```python
from build123d import *

# Parameters (mm, degrees)
SKETCH1_W           = 390
SKETCH1_H           = 88
BOSS_EXTRUDE1_DEPTH = 60
SKETCH2_R           = 13.520117845
BOSS_EXTRUDE2_DEPTH = 10
LPATTERN1_COUNT     = 6
LPATTERN1_PITCH     = 60


with BuildPart() as part:
    # Sketch1 → Boss-Extrude1 (new body)
    with BuildSketch(Plane.XY):
        with Locations((2.535, 19.375)):
            Rectangle(SKETCH1_W, SKETCH1_H)
    extrude(amount=BOSS_EXTRUDE1_DEPTH)

    # Sketch2 → Boss-Extrude2 (add)
    with BuildSketch(Plane.XY.offset(60)):
        with Locations((-142.569495457, 17.704999413)):
            Circle(SKETCH2_R)
    boss_extrude2 = extrude(amount=BOSS_EXTRUDE2_DEPTH)

    # LPattern1: Boss-Extrude2 ×6
    with Locations(*[(i * LPATTERN1_PITCH, 0, 0) for i in range(1, LPATTERN1_COUNT)]):
        add(boss_extrude2)


solid = part.part
```
For this review, take the finished solid that the model builds, in its own axes (mm). A direction names the side the tool comes from. Round coordinates to 2 decimals unless told otherwise and drop trailing zeros. Write each loop counter-clockwise with the first axis right and the second up, starting at its lowest first coordinate (ties: lowest second). Pieces come first, ordered by that corner, then holes. Notation, with made-up numbers: (56, 48.5) - (68, 48.5) arc R21 ccw to (68, 83.5) - close; hole circle Ø4 at (56.25, 60.25). An arc over 180 degrees is marked (long way). Answer as a JSON object with one key per item and string values.
1. We need section D-D on y = 23.5. Give the boundary of the cut face in (x, z) (3 decimals), then the cut area to 3 significant figures.
Response values:
{"outline": "(-192.465, 0) - (197.535, 0) - (197.535, 60) - (169.646, 60) - (169.646, 70) - (145.215, 70) - (145.215, 60) - (109.646, 60) - (109.646, 70) - (85.215, 70) - (85.215, 60) - (49.646, 60) - (49.646, 70) - (25.215, 70) - (25.215, 60) - (-10.354, 60) - (-10.354, 70) - (-34.785, 70) - (-34.785, 60) - (-70.354, 60) - (-70.354, 70) - (-94.785, 70) - (-94.785, 60) - (-130.354, 60) - (-130.354, 70) - (-154.785, 70) - (-154.785, 60) - (-192.465, 60) - close", "area": "24,900 mm2"}
2. To check wall thickness, follow line 1 along X through (y, z) = (25.5, 62); line 2 along Z through (x, y) = (127, 38). State the ranges of each line that lie inside material, in increasing order.
Response values:
{"line 1": "x = -153.62 to -131.52, -93.62 to -71.52, -33.62 to -11.52, 26.38 to 48.48, 86.38 to 108.48, 146.38 to 168.48", "line 2": "z = 0 to 60"}
3. We need section C-C on x = 147.5. Give the boundary of the cut face in (y, z) (3 decimals).
Response values:
{"outline": "(-24.625, 0) - (63.375, 0) - (63.375, 60) - (26.88, 60) - (26.88, 70) - (8.53, 70) - (8.53, 60) - (-24.625, 60) - close"}
4. Tool access review of faces 5 (the face through (94.5, 4.506, 64.93)), 6 (the face through (-192.465, 19, 30)): name each direction out of +Z, -Z, +X, -X, +Y, -Y from which nothing blocks a thin tool from reaching the whole face with its end or side.
Response values:
{"face 5": "+Z", "face 6": "+Z, -Z, -X, +Y, -Y"}
5. Draft analysis for pull direction X (two halves, no side actions). For faces 1 (the face through (-16.33, 5.71, 64.93)), 2 (the face through (-76.33, 5.71, 64.93)), 3 (the face through (197.535, 19, 30)), 4 (the face through (0, 20, 0)), state which applies: +X half, -X half, draft (parallel to the pull), parting line (faces both ways), or undercut.
Response values:
{"face 1": "undercut", "face 2": "undercut", "face 3": "+X half", "face 4": "draft"}
6. We need section A-A on y = -14.5. Give the boundary of the cut face in (x, z) (3 decimals), then the cut area to 3 significant figures.
Response values:
{"outline": "(-192.465, 0) - (197.535, 0) - (197.535, 60) - (-192.465, 60) - close", "area": "23,400 mm2"}
7. We need section B-B on x = -112.5. Give the boundary of the cut face in (y, z) (3 decimals).
Response values:
{"outline": "(-24.625, 0) - (63.375, 0) - (63.375, 60) - (-24.625, 60) - close"}
